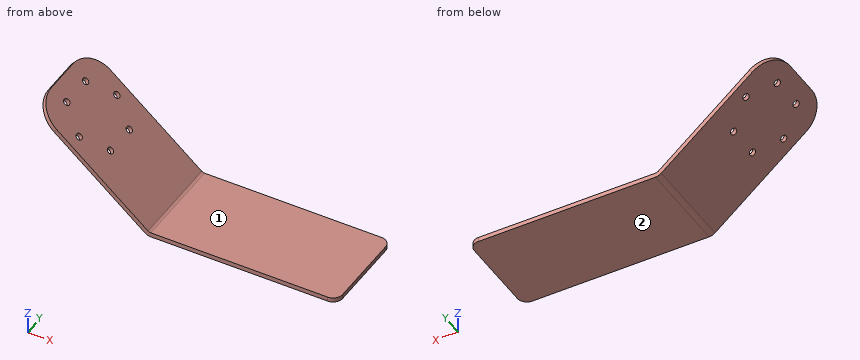
Autodesk Inventor part; units mm, degrees
ref_plane "YZ Plane" through (0, 0, 0) normal (1, 0, 0) x (0, 1, 0)
ref_plane "XZ Plane" through (0, 0, 0) normal (0, 1, 0) x (-1, 0, 0)
ref_plane "XY Plane" through (0, 0, 0) normal (0, 0, 1) x (1, 0, 0)
sketch "Sketch1" plane through (0, 0, 0) normal (0, 0, 1) x (1, 0, 0)
  line L0 (63.5, -31.75) -> (-63.5, -31.75)
  line L1 (-63.5, -31.75) -> (-63.5, 31.75)
  line L2 (-63.5, 31.75) -> (63.5, 31.75)
  line L3 (63.5, 31.75) -> (63.5, -31.75)
  line L4 (63.5, -31.75) -> (-63.5, 31.75) construction
  line L5 (-63.5, -31.75) -> (63.5, 31.75) construction
  point P0 (0, 0)
  dimension "d0" = 63.5
  dimension "d1" = 127
extrude "Plate1" add sketch "Sketch1" along normal blind 3.048
sketch "Sketch2" plane through (-63.5, -31.75, 3.048) normal (-0.6427876, 0, -0.7660444) x (0, -1, 0)
  line L0 (-63.5, 0) -> (0, 0)
  line L1 (0, 0) -> (0, 100.4906)
  line L2 (0, 100.4906) -> (-63.5, 100.4906)
  line L3 (-63.5, 100.4906) -> (-63.5, 0)
edge flange "Flange1" height 101.6 angle 40 thickness 3.048 bend radius 3.048 thickness toward (-0.6427876, 0, -0.7660444) relief tear relief width 3.048 relief depth 1.524 edges at (-63.5, 0, 3.048) wall of the first edge with corners at (-63.5, 31.75, 3.048) (-63.5, -31.75, 3.048) (-140.4803, -31.75, 67.6421) (-140.4803, 31.75, 67.6421)
bend "Bend1"
corner "Corner1"
sketch "Sketch3" plane through (-142.4395, -31.75, 65.3072) normal (-0.6427876, 0, -0.7660444) x (-0.7660444, 0, 0.6427876)
  circle A0 centre (-31.75, 31.75) radius 22.225 construction
  line L0 (-99.3812, 63.5) -> (0, 63.5) construction
  line L1 (0, 63.5) -> (0, 0) construction
  point P0 (-151.0937, 31.75)
  point P1 (-49.6906, 63.5)
  point P2 (-31.75, 53.975)
  point P3 (-50.9974, 42.8625)
  point P4 (-50.9974, 20.6375)
  point P5 (-31.75, 9.525)
  point P6 (-12.5026, 20.6375)
  point P7 (-12.5026, 42.8625)
  dimension "d13" = 44.45
  dimension "d16" = 360
  dimension "d25" = 31.75
hole "Hole1" at (-118.1176, 22.225, 44.8987) at (-103.3732, 11.1125, 32.5267) at (-103.3732, -11.1125, 32.5267) at (-118.1176, -22.225, 44.8987) at (-132.862, -11.1125, 57.2707) at (-132.862, 11.1125, 57.2707) direction (0.6427876, 0, 0.7660444) diameter 4.4958 depth 3.048 tip angle 118
fillet "Fillet1" radius 19.05 2 edges at (-141.4599, -31.75, 66.4747) (-141.4599, 31.75, 66.4747)
fillet "Fillet2" radius 6.35 2 edges at (63.5, 31.75, 1.524) (63.5, -31.75, 1.524)
equation "\"d23\" = Thickness"
equation "\"d2\" = Thickness"
equation "\"d3\" = BendReliefWidth"
equation "\"d4\" = BendReliefDepth"
equation "\"d5\" = MinimumRemnant"
equation "\"d6\" = TransitionRadius"
equation "\"d9\" = BendRadius"
equation "\"d10\" = CornerReliefSize"
equation "\"d11\" = GapSize"
equation "\"d12\" = JacobiRadiusSize"
equation "\"BendRadius\" = Thickness"
equation "\"BendReliefWidth\" = Thickness"
equation "\"BendReliefDepth\" = 0.5 * Thickness"
equation "\"CornerReliefSize\" = 4 * Thickness"
equation "\"MinimumRemnant\" = 2 * Thickness"
equation "\"TransitionRadius\" = BendRadius"
equation "\"JacobiRadiusSize\" = BendRadius"
equation "\"GapSize\" = Thickness"
properties part number "CL7-023" material "Polycarbonate, Smoke"
Geometry check sheet. Reference: the model listing, model coordinates, mm. Face numbers are marked on the shaded views. A direction names the side the tool comes from. Give positions to 0.01 mm unless a question says otherwise; leave off trailing zeros. Write each loop counter-clockwise with the first axis right and the second up, starting at its lowest first coordinate (ties: lowest second). Pieces come first, ordered by that corner, then holes. Notation, with made-up numbers: (12, -21.75) -> (41, -21.75) arc R17 ccw to (41, -17.75) -> close; hole circle Ø2 at (-14.75, 55.25). An arc over 180 degrees is marked (long way). One line per question, with ' | ' between items.
Item 1: Sectioned sample at D-D, the plane y = 16.5. Record the boundary of the cut face in (x, z).
Determined:
outline: (-142.15, 65.06) -> (-66.31, 1.43) arc R6.1 ccw to (-62.39, 0) -> (63.5, 0) -> (63.5, 3.05) -> (-62.39, 3.05) arc R3.05 cw to (-64.35, 3.76) -> (-140.19, 67.4) -> close
Item 2: Sectioned sample at B-B, the plane x = 11. Record the boundary of the cut face in (y, z).
Determined:
outline: (-31.75, 0) -> (31.75, 0) -> (31.75, 3.05) -> (-31.75, 3.05) -> close
Item 3: Sectioned sample at A-A, the plane y = -6.5. Record the boundary of the cut face in (x, z).
Determined:
outline: (-142.44, 65.31) -> (-66.31, 1.43) arc R6.1 ccw to (-62.39, 0) -> (63.5, 0) -> (63.5, 3.05) -> (-62.39, 3.05) arc R3.05 cw to (-64.35, 3.76) -> (-140.48, 67.64) -> close
Item 4: Depth check by flat-ended pin: pin 1 (8 mm diameter, centred on y = -6.5, z = 51.5, fed in from +X); pin 2 (10 mm diameter, centred on x = -22.5, y = 4.5, fed in from -Z); pin 3 (6 mm diameter, centred on y = -1.5, z = 16, fed in from +X); pin 4 (10 mm diameter, centred on y = 13.5, z = 9, fed in from +X). Enter the tip coordinate at first touch or a pass-through.
Determined:
pin 1: x = -116.48 | pin 2: z = 0 | pin 3: x = -75.36 | pin 4: x = -64.63
Item 5: Access from +Z, -Z, +X, -X, +Y, -Y to the whole of each face (thin tool, end or side, straight path). Record for the marked faces 1 and 2.
Determined:
face 1: +Z, +X, +Y, -Y | face 2: -Z, +X, -X, +Y, -Y
Item 6: Sectioned sample at C-C, the plane z = 19. Record the boundary of the cut face in (x, y), plus the area to 3 significant figures.
Determined:
outline: (-87.25, -31.75) -> (-82.51, -31.75) -> (-82.51, 31.75) -> (-87.25, 31.75) -> close | area: 301 mm^2
Item 7: Scan lines: line 1 along Z through (x, y) = (40, -5); line 2 along Z through (x, y) = (-77, -13.5); line 3 along X through (y, z) = (-8, 30). Record each from-to range of solid material in increasing order.
Determined:
line 1: 0 to 3.05 | line 2: 10.4 to 14.38 | line 3: -100.36 to -95.62
